Could you check a few things on this drawing? It's one solid part, dimensions in mm from its lowest x, y, z. Give positions to 0.01 mm unless a question says otherwise; leave off trailing zeros. Loops run counter-clockwise (first coordinate to the right, second up) from the corner with the lowest first, then second, coordinate; pieces in that order, holes last. Notation, with made-up numbers: M -28,64.25 L 10,64.25 A16 cw 10,95.25 Z; hole C -27,-32.75 d10. An arc over 180 degrees is marked long. Answer as CSV lines item,"result". Start each with the question number.
Item 1: If I drill on line 1 along Y through (x, z) = (4.3, 83); line 2 along Z through (x, y) = (3.4, 11), over which ranges is the centre line in solid material (lowest first)? Write a range as from..to.
Item 2: I want a section at B-B on z = 108.5. List the corners of the cut face in (x, y) for me.
Item 3: I want a section at A-A on y = 57. List the corners of the cut face in (x, z) for me.
Item 4: Will these pins go through, and if not, where does the flat tip stop? P1, Ø1.5, axis at x = 4, z = 96, coming from the -Y side; P2, Ø2.5, axis at x = 3.5, y = 9.5, coming from the -Z side; P3, Ø2.5, axis at x = 1.5, z = 3.5, coming from the -Y side (3 decimals); P4, Ø1.6, axis at x = 3, z = 2.5, coming from the +Y side (3 decimals).
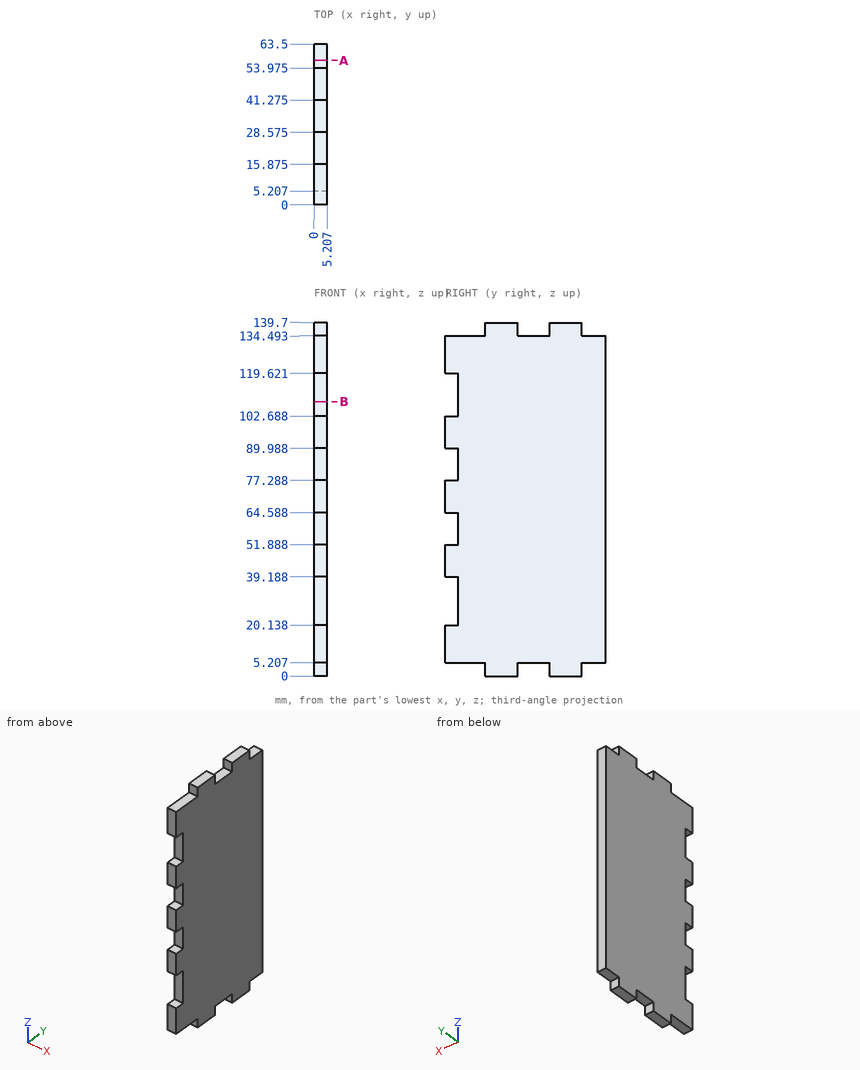
Result:
1,line 1,"5.21..63.5"
1,line 2,"5.21..134.49"
2,outline,"M 0,5.21 L 5.21,5.21 L 5.21,63.5 L 0,63.5 Z"
3,outline,"M 0,5.21 L 5.21,5.21 L 5.21,134.49 L 0,134.49 Z"
4,P1,"y = 0"
4,P2,"z = 5.21"
4,P3,"y = 15.875"
4,P4,"y = 53.975"
